Design review of the part built by this model. Coordinates are the model's own, in mm. A direction names the side the tool comes from. Round coordinates to 2 decimals unless told otherwise and drop trailing zeros. Order: outer loops, then holes, each group sorted by start corner. A loop starts at its lowest first (then second) coordinate and runs counter-clockwise, first axis right, second up. Notation, with made-up numbers: M 33.5,70 L 41.5,70 A27 ccw 41.5,103 Z; hole C -13.5,-12.5 d10. An arc over 180 degrees is marked long. Write each question's results on one line, items separated by ' | '. Start each with the question number.
Item 1: Take a section at B-B, the plane y = 0. Write out the cut boundary in (x, z).
Item 2: Wall thickness on line 1 (Y direction, x = 1, z = 7.75); line 2 (Y direction, x = 1, z = 0.5); line 3 (X direction, y = -22.5, z = 3.75): over which ranges is each line inside the solid? List them lowest first. Write a range as [from, to].
Item 3: Clearance check with flat-ended pins moving along their axes: pin 1 (1 mm diameter, centred on y = 29.5, z = 7, fed in from +X); pin 2 (2 mm diameter, centred on x = 23.5, y = -64, fed in from +Z); pin 3 (1.5 mm diameter, centred on x = -3.5, y = 33.5, fed in from -Z); pin 4 (1.4 mm diameter, centred on x = 23, y = 44, fed in from +Z). State where each tip first meets the part, or that it passes through.
Item 4: Machinability: for faces 1 (the flat face through (-19.95, -36, 6)), 2 (the flat face through (15, -15, 10)), 3 (the cylindrical face through (-3.47, -15.62, 4.03)), which of the approach directions +Z, -Z, +X, -X, +Y, -Y give a long, thin tool a straight path to every point of the face, cutting with its end or side? Answer none if there is none.
Item 5: Take a section at C-C, the plane y = -35. Write out the cut boundary in (x, z).
Item 6: Take a section at A-A, the plane x = 0. Write out the cut boundary in (y, z), plus the area to 3 significant figures.
```python
from build123d import *

# Parameters (mm, degrees)
F1_DEPTH      = 64.75
F2_W          = 1.8
F2_H          = 125.7
F3_DEPTH      = 1
F4_R          = 20
F5_DEPTH      = 4
F6_R          = 16
F7_DEPTH      = 4
F8_R          = 14
F9_DEPTH      = 2.001
F10_T         = 2
F10_T3_DEPTH  = 5.9
F10_T5_DEPTH  = 5
F10_T7_DEPTH  = 5.8
F10_T9_DEPTH  = 129.7
F10_T11_DEPTH = 5.9
F10_T13_DEPTH = 5.8
F11_W         = 1.1
F11_H         = 6.75
F12_DEPTH     = 1.9


# Not quite as in the source:
# - a pattern or mirror of a feature is missing from the dataset's text; its kind, count and spacing are read off the source's solid
# - a shell that OpenCascade refuses in one call is made with other operations: the cavity is built on its own and cut out


with BuildPart() as f1:
    # F0 (on Front) → F1 (new body, symmetric)
    with BuildSketch(Plane.XZ):
        Polygon((-23.75, 7.75), (-23.75, 0), (23.75, 0), (23.75, 7.75), (21.95, 7.75), (21.95, 10), (-21.95, 10), (-21.95, 7.75), align=None)
    extrude(amount=F1_DEPTH, both=True)

    # F2 (on face) → F3 (cut)
    with BuildSketch(Plane.XY.offset(7.75)):
        with Locations((22.85, 0)):
            Rectangle(F2_W, F2_H)
    f3 = extrude(amount=-F3_DEPTH, mode=Mode.SUBTRACT)

    # F3_copies: F3 across plane
    add(f3.mirror(Plane(origin=(0, 0, 0), x_dir=(0, 0, -1), z_dir=(-1, 0, 0))), mode=Mode.SUBTRACT)

    # F4 (on face) → F5 (cut)
    with BuildSketch(Plane.XY.offset(10)):
        Circle(F4_R)
    extrude(amount=-F5_DEPTH, mode=Mode.SUBTRACT)

    # F6 (on face) → F7 (cut)
    with BuildSketch(Plane.XY.offset(6)):
        Circle(F6_R)
    extrude(amount=-F7_DEPTH, mode=Mode.SUBTRACT)

    # F8 (on face) → F9 (cut, through all)
    with BuildSketch(Plane.XY.offset(2)):
        Circle(F8_R)
    extrude(amount=-F9_DEPTH, mode=Mode.SUBTRACT)

    # F10: shell of thickness 2, made by hand


with BuildPart() as f10_core1:
    # F10_t2: copy of F1
    add(f1.part)

    # the walls: a layer under each face that stays
    f10_faces = [f10_core1.faces().sort_by_distance(p)[0] for p in [
        (-23.75, 0, 3.875),
        (-22.85, 63.8, 7.75),
        (-22.85, 62.85, 7.25),
        (-22.85, 0, 6.75),
        (-22.85, -62.85, 7.25),
        (-22.85, -63.8, 7.75),
        (0, -64.75, 5),
        (0, 64.75, 5),
        (-21.95, 0, 8.375),
        (23.75, 0, 3.875),
        (22.85, -63.8, 7.75),
        (21.95, 0, 8.375),
        (14.6333333333, 43.1666666667, 10),
        (-14, 0, 1),
        (22.85, 63.8, 7.75),
        (22.85, -62.85, 7.25),
        (22.85, 0, 6.75),
        (22.85, 62.85, 7.25),
        (-20, 0, 8),
        (-10.6666666667, -10.6666666667, 2),
        (-13.3333333333, -13.3333333333, 6),
        (-16, 0, 4),
    ]]
    thicken(f10_faces, amount=-F10_T, mode=Mode.SUBTRACT)

    # F10_s4 → F10_t3 (cut)
    with BuildSketch(Plane.XZ.offset(-66.75)):
        Polygon((-21.97, 7.77), (-21.95, 5.75), (-19.95, 5.75), (-19.95, 7.75), align=None)
        Polygon((21.97, 7.77), (19.95, 7.75), (19.95, 5.75), (21.95, 5.75), align=None)
    extrude(amount=F10_T3_DEPTH, mode=Mode.SUBTRACT)

    # F10_s6 → F10_t5 (cut)
    with BuildSketch(Plane.XY.offset(4.75)):
        Polygon((-21.97, 62.83), (-21.95, 64.85), (-19.95, 64.85), (-19.95, 62.85), align=None)
        Polygon((-21.97, -62.83), (-21.95, -64.85), (-19.95, -64.85), (-19.95, -62.85), align=None)
        Polygon((21.97, -62.83), (19.95, -62.85), (19.95, -64.85), (21.95, -64.85), align=None)
        Polygon((21.97, 62.83), (19.95, 62.85), (19.95, 64.85), (21.95, 64.85), align=None)
    extrude(amount=F10_T5_DEPTH, mode=Mode.SUBTRACT)

    # F10_s8 → F10_t7 (cut)
    with BuildSketch(Plane.YZ.offset(-25.75)):
        Polygon((62.83, 6.77), (64.85, 6.75), (64.85, 4.75), (62.85, 4.75), align=None)
        Polygon((-62.83, 6.77), (-62.85, 4.75), (-64.85, 4.75), (-64.85, 6.75), align=None)
    extrude(amount=F10_T7_DEPTH, mode=Mode.SUBTRACT)

    # F10_s10 → F10_t9 (cut)
    with BuildSketch(Plane.XZ.offset(-64.85)):
        Polygon((-21.97, 6.77), (-21.95, 4.75), (-19.95, 4.75), (-19.95, 6.75), align=None)
        Polygon((21.97, 6.77), (19.95, 6.75), (19.95, 4.75), (21.95, 4.75), align=None)
    extrude(amount=F10_T9_DEPTH, mode=Mode.SUBTRACT)

    # F10_s12 → F10_t11 (cut)
    with BuildSketch(Plane.XZ.offset(60.85)):
        Polygon((-21.97, 7.77), (-21.95, 5.75), (-19.95, 5.75), (-19.95, 7.75), align=None)
        Polygon((21.97, 7.77), (21.95, 5.75), (19.95, 5.75), (19.95, 7.75), align=None)
    extrude(amount=F10_T11_DEPTH, mode=Mode.SUBTRACT)

    # F10_s14 → F10_t13 (cut)
    with BuildSketch(Plane.YZ.offset(19.95)):
        Polygon((-62.83, 6.77), (-64.85, 6.75), (-64.85, 4.75), (-62.85, 4.75), align=None)
        Polygon((62.83, 6.77), (62.85, 4.75), (64.85, 4.75), (64.85, 6.75), align=None)
    extrude(amount=F10_T13_DEPTH, mode=Mode.SUBTRACT)

    # F10_s15 → F10_t16 (revolve, cut)
    with BuildSketch(Plane.XZ):
        Polygon((19.98, 6.02), (22, 6), (22, 4), (20, 4), align=None)
    revolve(axis=Axis((0, 0, 6), (0, 0, 1)), mode=Mode.SUBTRACT)

    # F10_s17 → F10_t18 (revolve, cut)
    with BuildSketch(Plane.XZ):
        Polygon((15.98, 2.02), (16, 0), (18, 0), (18, 2), align=None)
    revolve(axis=Axis((0, 0, 2), (0, 0, 1)), mode=Mode.SUBTRACT)


with BuildPart() as f1_1:
    add(f1.part)

    # what is left inside the walls is the cavity
    f10_cavity = [f10_core1.part.solids().sort_by_distance(p)[0] for p in [
        (0, 20.916667, 0.02),
    ]]
    add(f10_cavity, mode=Mode.SUBTRACT)

    # F11 (on face) → F12 (cut)
    with BuildSketch(Plane.YZ.offset(23.75)):
        with Locations((5.9, 3.375)):
            Rectangle(F11_W, F11_H)
    extrude(amount=-F12_DEPTH, mode=Mode.SUBTRACT)


solid = f1_1.part
```
Results list:
1) outline: M -23.75,0 L -21.75,0 L -21.75,4 L -18,4 L -18,0 L -14,0 L -14,2 L -16,2 L -16,6 L -20,6 L -20,10 L -21.95,10 L -21.95,6.75 L -23.75,6.75 Z; M 14,0 L 18,0 L 18,4 L 21.75,4 L 21.75,0 L 23.75,0 L 23.75,6.75 L 21.95,6.75 L 21.95,10 L 20,10 L 20,6 L 16,6 L 16,2 L 14,2 Z
2) line 1: [-64.75, -62.75], [-21.98, -19.97], [19.97, 21.98], [62.75, 64.75] | line 2: [-64.75, -62.75], [-17.97, -13.96], [13.96, 17.97], [62.75, 64.75] | line 3: [-23.75, -21.75], [21.75, 23.75]
3) pin 1: x = 23.75 | pin 2: z = 7.75 | pin 3: z = 8 | pin 4: z = 6.75
4) face 1: -Z | face 2: +Z, +X, -X, +Y, -Y | face 3: +Z
5) outline: M -23.75,0 L -21.75,0 L -21.75,4.75 L -19.95,4.75 L -19.95,8 L 19.95,8 L 19.95,4.75 L 21.75,4.75 L 21.75,0 L 23.75,0 L 23.75,6.75 L 21.95,6.75 L 21.95,10 L -21.95,10 L -21.95,6.75 L -23.75,6.75 Z
6) outline: M -64.75,0 L -62.75,0 L -62.75,8 L -22,8 L -22,4 L -18,4 L -18,0 L -14,0 L -14,2 L -16,2 L -16,6 L -20,6 L -20,10 L -64.75,10 Z; M 14,0 L 18,0 L 18,4 L 22,4 L 22,8 L 62.75,8 L 62.75,0 L 64.75,0 L 64.75,10 L 20,10 L 20,6 L 16,6 L 16,2 L 14,2 Z | area: 267 mm²
